Work out the finished part from the listing and answer in its coordinate system (mm). A direction names the side the tool comes from. Coordinates: 2 decimals unless noted, no trailing zeros. Loops run counter-clockwise (first coordinate to the right, second up) from the corner with the lowest first, then second, coordinate; pieces in that order, holes last. Notation, with made-up numbers: (-33.5, 52.5) -> (-10.5, 52.5) arc R14 ccw to (-10.5, 78.5) -> close; hole circle Ø2 at (43.5, 77.25). An arc over 180 degrees is marked (long way). One line per question, with ' | ' between items.
```python
from build123d import *

# Parameters (mm, degrees)
BOSS_EXTRUDE1_DEPTH = 35
CUT_EXTRUDE1_DEPTH  = 89.600225733
SKETCH3_R           = 4.25
CUT_EXTRUDE2_DEPTH  = 78.781745931
CUT_EXTRUDE6_DEPTH  = 35
CUT_EXTRUDE7_REACH  = 82.156
SKETCH5_R           = 2


with BuildPart() as part:
    # Sketch1 → Boss-Extrude1 (new body)
    with BuildSketch(Plane(origin=(0, 0, 0), x_dir=(1, 0, 0), z_dir=(0, 1, 0))):
        Polygon((-60, 15), (60, 15), (60, -5), (17.5, -5), (17.5, -40), (-17.5, -40), (-17.5, -5), (-60, -5), align=None)
    extrude(amount=BOSS_EXTRUDE1_DEPTH)

    # Sketch2 → Cut-Extrude1 (cut, through all)
    with BuildSketch(Plane.XY.offset(40)):
        with BuildLine():
            Line((3, 28.75), (-3, 28.75))
            Line((-3, 28.75), (-3, 27.039392014))
            ThreePointArc((-3, 27.039392014), (0, 27.5), (3, 27.039392014))
            Line((3, 27.039392014), (3, 28.75))
        make_face()
        with BuildLine():
            ThreePointArc((3, 27.039392014), (0, 27.5), (-3, 27.039392014))
            Line((-3, 27.039392014), (3, 27.039392014))
        make_face()
        with BuildLine():
            Line((3, 27.039392014), (-3, 27.039392014))
            ThreePointArc((-3, 27.039392014), (-5.916079783, 9.437742252), (10, 17.5))
            ThreePointArc((10, 17.5), (8.062257748, 23.416079783), (3, 27.039392014))
        make_face()
    extrude(amount=-CUT_EXTRUDE1_DEPTH, mode=Mode.SUBTRACT)

    # Sketch3 → Cut-Extrude2 (cut, through all)
    with BuildSketch(Plane.XY.offset(5)):
        with Locations((-50, 17.5)):
            Circle(SKETCH3_R)
        with Locations((-32, 17.5)):
            Circle(SKETCH3_R)
        with Locations(Location((32, 17.5, 0), (0, 0, 180))):
            Circle(SKETCH3_R)
        with Locations(Location((50, 17.5, 0), (0, 0, 180))):
            Circle(SKETCH3_R)
    extrude(amount=-CUT_EXTRUDE2_DEPTH, mode=Mode.SUBTRACT)

    # Sketch4 → Cut-Extrude6 (cut)
    with BuildSketch(Plane.XY.offset(40)):
        with BuildLine():
            Line((0, 35), (-17.5, 35))
            Line((-17.5, 35), (-17.5, 17.5))
            ThreePointArc((-17.5, 17.5), (-12.374368671, 29.874368671), (0, 35))
        make_face()
        with BuildLine():
            Line((17.5, 35), (0, 35))
            ThreePointArc((0, 35), (12.374368671, 29.874368671), (17.5, 17.5))
            Line((17.5, 17.5), (17.5, 35))
        make_face()
        with BuildLine():
            Line((17.5, 0), (17.5, 17.5))
            ThreePointArc((17.5, 17.5), (12.374368681, 5.12563134), (3e-08, 0))
            Line((3e-08, 0), (17.5, 0))
        make_face()
        with BuildLine():
            ThreePointArc((3e-08, 0), (-12.37436866, 5.125631319), (-17.5, 17.5))
            Line((-17.5, 17.5), (-17.5, 0))
            Line((-17.5, 0), (3e-08, 0))
        make_face()
    extrude(amount=-CUT_EXTRUDE6_DEPTH, mode=Mode.SUBTRACT)

    # Sketch5 → Cut-Extrude7 (cut, up to next)
    with BuildSketch(Plane(origin=(0, 35, 0), x_dir=(1, 0, 0), z_dir=(0, 1, 0)), mode=Mode.PRIVATE) as cut_extrude7_sk1:
        with Locations(Location((0, -32.5, 0), (0, 0, 270))):
            Circle(SKETCH5_R)
    cut_extrude7_tool1 = extrude(cut_extrude7_sk1.sketch, amount=-CUT_EXTRUDE7_REACH, mode=Mode.PRIVATE) & part.part
    # Sketch5 → Cut-Extrude7 (cut, up to next)
    with BuildSketch(Plane(origin=(0, 35, 0), x_dir=(1, 0, 0), z_dir=(0, 1, 0)), mode=Mode.PRIVATE) as cut_extrude7_sk2:
        with Locations(Location((0, -11.5, 0), (0, 0, 270))):
            Circle(SKETCH5_R)
    cut_extrude7_tool2 = extrude(cut_extrude7_sk2.sketch, amount=-CUT_EXTRUDE7_REACH, mode=Mode.PRIVATE) & part.part
    add(cut_extrude7_tool1.solids().sort_by_distance((0, 35, 32.5))[0], mode=Mode.SUBTRACT)
    add(cut_extrude7_tool2.solids().sort_by_distance((0, 35, 11.5))[0], mode=Mode.SUBTRACT)


solid = part.part
```
1) Find section D-D (x = -12.5). Write down the section's boundary in (y, z), plus the area to 3 significant figures.
Check values:
outline: (0, -15) -> (35, -15) -> (35, 5) -> (29.75, 5) -> (29.75, 40) -> (5.25, 40) -> (5.25, 5) -> (0, 5) -> close | area: 1,560 mm^2
2) Find section A-A (z = -5). Write down the section's boundary in (x, y).
Check values:
outline: (-60, 0) -> (60, 0) -> (60, 35) -> (-60, 35) -> close; hole circle Ø8.5 at (-50, 17.5); hole circle Ø8.5 at (-32, 17.5); hole (-3, 27.04) arc R10 ccw (long way) to (3, 27.04) -> (3, 28.75) -> (-3, 28.75) -> close; hole circle Ø8.5 at (32, 17.5); hole circle Ø8.5 at (50, 17.5)
3) For faces 1 (the face through (-1, 29, -15)), 2 (the face through (2, 28.75, 13)), determine the directions among +Z, -Z, +X, -X, +Y, -Y from which every point of the face is accessible in a straight line to the end or side of a thin tool.
Check values:
face 1: -Z, +X, -X, +Y, -Y | face 2: +Z, -Z
4) Find section C-C (z = 6.5). Write down the section's boundary in (x, y).
Check values:
outline: circle Ø35 at (0, 17.5); hole (-3, 27.04) arc R10 ccw (long way) to (3, 27.04) -> (3, 28.75) -> (-3, 28.75) -> close
5) Find section B-B (x = 32). Write down the section's boundary in (y, z), plus the area to 3 significant figures.
Check values:
outline: (0, -15) -> (13.25, -15) -> (13.25, 5) -> (0, 5) -> close; (21.75, -15) -> (35, -15) -> (35, 5) -> (21.75, 5) -> close | area: 530 mm^2
6) Find the intervals of material crossed by line 1 along Y through (x, z) = (-50, -4); line 2 along X through (y, z) = (17, -5); line 3 along Z through (x, y) = (-37.5, 25), in increasing order.
Check values:
line 1: y = 0 to 13.25, 21.75 to 35 | line 2: x = -60 to -54.22, -45.78 to -36.22, -27.78 to -9.99, 9.99 to 27.78, 36.22 to 45.78, 54.22 to 60 | line 3: z = -15 to 5
7) The mould has two halves that part along Z. Classify faces 3 (the face through (36, 22, 5)), 4 (the face through (-0.766, 31.919, 34.347)), 5 (the face through (1, 35, -5)), 6 (the face through (-1.2, 31.9, 9.9)): released by +Z, released by -Z, zero draft, split by the parting line, or undercut.
Check values:
face 3: released by +Z | face 4: undercut | face 5: zero draft | face 6: undercut
8) Flat-ended cylindrical pins translate along their axes: pin 1 (10.5 mm diameter, centred on x = -41, y = 18, fed in from +Z); pin 2 (7 mm diameter, centred on x = -32, y = 17.5, fed in from -Z); pin 3 (10 mm diameter, centred on x = -9.5, y = 20, fed in from +Z); pin 4 (5 mm diameter, centred on x = -12, z = 27, fed in from +Y). Find the tip coordinate at first contact, or state that the pin passes through.
Check values:
pin 1: stops at z = 5 | pin 2: passes through | pin 3: stops at z = 40 | pin 4: stops at y = 32.2
